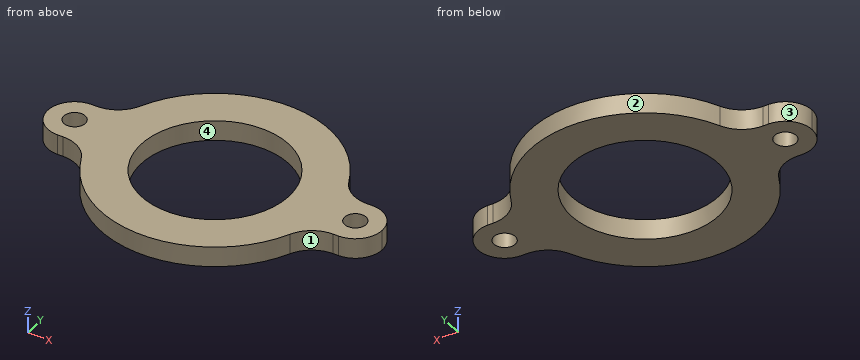
from build123d import *

# Parameters (mm, degrees)
ESBO_O1_R                = 11
ESBO_O1_R_2              = 1.6
RESSALTO_EXTRUS_O1_DEPTH = 3
FILETE2_R                = 5
FILETE3_R                = 4


with BuildPart() as part:
    # Esboço1 → Ressalto-extrusão1 (new body)
    with BuildSketch(Plane.XY):
        with BuildLine():
            Line((-25, 4), (-16.625582697, 4))
            ThreePointArc((-16.625582697, 4), (0, 17.1), (16.625582697, 4))
            Line((16.625582697, 4), (25, 4))
            Line((25, 4), (25, -4))
            Line((25, -4), (16.625582697, -4))
            ThreePointArc((16.625582697, -4), (0, -17.1), (-16.625582697, -4))
            Line((-16.625582697, -4), (-25, -4))
            Line((-25, -4), (-25, 4))
        make_face()
        Circle(ESBO_O1_R, mode=Mode.SUBTRACT)
        with Locations((-21, 0)):
            Circle(ESBO_O1_R_2, mode=Mode.SUBTRACT)
        with Locations((21, 0)):
            Circle(ESBO_O1_R_2, mode=Mode.SUBTRACT)
    extrude(amount=RESSALTO_EXTRUS_O1_DEPTH)

    # Filete2
    filete2_edges = [part.edges().sort_by_distance(p)[0] for p in [
        (-16.625582697, 4, 1.5),
        (16.625582697, 4, 1.5),
        (16.625582697, -4, 1.5),
        (-16.625582697, -4, 1.5),
    ]]
    fillet(filete2_edges, radius=FILETE2_R)

    # Filete3
    filete3_edges = [part.edges().sort_by_distance(p)[0] for p in [
        (25, -4, 1.5),
        (25, 4, 1.5),
        (-25, -4, 1.5),
        (-25, 4, 1.5),
    ]]
    fillet(filete3_edges, radius=FILETE3_R - 0.0001)  # a hair under: the kernel refuses the full size


solid = part.part
CAD build for the part. Positions are in the model's coordinates, mm. Face numbers are marked on the shaded views. Coordinates: 2 decimals unless noted, no trailing zeros. Order: outer loops, then holes, each group sorted by start corner. A loop starts at its lowest first (then second) coordinate and runs counter-clockwise, first axis right, second up.
Item 1: Band-saw the part on D-D on y = -14. List the corners of the cut face in (x, z), plus the area to 3 significant figures.
Check sheet entries:
outline: (-9.82, 0) - (9.82, 0) - (9.82, 3) - (-9.82, 3) - close
area: 58.9 mm2
Item 2: Band-saw the part on C-C on y = 3. List the corners of the cut face in (x, z), plus the area to 3 significant figures.
Check sheet entries:
outline: (-23.65, 0) - (-10.58, 0) - (-10.58, 3) - (-23.65, 3) - close; (10.58, 0) - (23.65, 0) - (23.65, 3) - (10.58, 3) - close
area: 78.4 mm2
Item 3: Pin check, flat tips, straight feed: pin 1 Ø0.7 at (x, z) = (-20.5, 1) entering from +Y; pin 2 Ø0.9 at (x, z) = (-20.5, 2) entering from -Y; pin 3 Ø1 at (x, z) = (-18, 2) entering from -Y; pin 4 Ø3 at (x, y) = (-10.5, 1.5) entering from -Z. Stop position of each tip, or through.
Check sheet entries:
pin 1: stops at y = 4
pin 2: stops at y = -4
pin 3: stops at y = -4.78
pin 4: stops at z = 0
Item 4: Band-saw the part on B-B on x = -0.5. List the corners of the cut face in (y, z), plus the area to 3 significant figures.
Check sheet entries:
outline: (-17.09, 0) - (-10.99, 0) - (-10.99, 3) - (-17.09, 3) - close; (10.99, 0) - (17.09, 0) - (17.09, 3) - (10.99, 3) - close
area: 36.6 mm2
Item 5: Drill centre lines: L1, parallel to Y at x = -21, z = 0.8; L2, parallel to Y at x = 0, z = 1.8; L3, parallel to X at y = -8, z = 0.8. Where is each one in solid material? Low to high.
Check sheet entries:
L1: y = -4 to -1.6, 1.6 to 4
L2: y = -17.1 to -11, 11 to 17.1
L3: x = -15.11 to -7.55, 7.55 to 15.11
Item 6: Two-plate mould, pull along X, no slides. Class the marked faces 1, 2, 3 and 4: +X half, -X half, draft (parallel to the pull), parting line (faces both ways), or undercut.
Check sheet entries:
face 1: +X half
face 2: parting line
face 3: -X half
face 4: undercut
Item 7: Band-saw the part on A-A on z = 2.2. Give the number of separate pieces and of enclosed holes in the cut face, plus the area to 3 significant figures.
Check sheet entries:
separate pieces: 1
enclosed holes: 3
area: 646 mm2
